Can you work these out from the model? Positions are in its coordinate system, mm. A direction names the side the tool comes from. Round coordinates to 2 decimals unless told otherwise and drop trailing zeros. Loops run counter-clockwise (first coordinate to the right, second up) from the corner with the lowest first, then second, coordinate; pieces in that order, holes last. Notation, with made-up numbers: (76, 34) -> (109, 34) arc R19 cw to (109, 60) -> close; hole circle Ø7 at (-26.75, 6.25). An arc over 180 degrees is marked (long way). Use a Markdown table: item, result.
from build123d import *

# Parameters (mm, degrees)
SKETCH1_W            = 229
SKETCH1_H            = 120
BOSS_EXTRUDE1_DEPTH  = 15
SKETCH2_W            = 20.632503002
SKETCH2_H            = 53.730004003
BOSS_EXTRUDE2_DEPTH  = 15
CUT_EXTRUDE1_REACH   = 239.205
SKETCH3_W            = 61.75
SKETCH3_H            = 25
CUT_EXTRUDE2_REACH   = 239.205
SKETCH4_W            = 61.75
SKETCH4_H            = 25
CUT_EXTRUDE5_REACH   = 239.205
SKETCH10_W           = 61.75
SKETCH10_H           = 25
CUT_EXTRUDE3_REACH   = 239.205
SKETCH5_R            = 7.5
SKETCH9_R            = 6.25
CUT_EXTRUDE4_DEPTH   = 5
LPATTERN2_COUNT      = 4
LPATTERN2_PITCH      = 69.677
LPATTERN2_COUNT_DIR2 = 2
LPATTERN2_PITCH_DIR2 = 100
M5_TAPPED_HOLE1_D    = 4.2
CUT_EXTRUDE6_REACH   = 239.205
SKETCH14_R           = 3.1


with BuildPart() as part:
    # Sketch1 → Boss-Extrude1 (new body)
    with BuildSketch(Plane(origin=(0, 0, 0), x_dir=(1, 0, 0), z_dir=(0, 1, 0))):
        with Locations((-114.5, 0)):
            Rectangle(SKETCH1_W, SKETCH1_H)
    extrude(amount=-BOSS_EXTRUDE1_DEPTH)

    # Sketch2 → Boss-Extrude2 (add)
    with BuildSketch(Plane(origin=(0, 0, 0), x_dir=(1, 0, 0), z_dir=(0, 1, 0))):
        with Locations((10.316251501, 33.134997999)):
            Rectangle(SKETCH2_W, SKETCH2_H)
    extrude(amount=-BOSS_EXTRUDE2_DEPTH)

    # Sketch3 → Cut-Extrude1 (cut, up to next)
    with BuildSketch(Plane(origin=(0, 0, 0), x_dir=(1, 0, 0), z_dir=(0, 1, 0)), mode=Mode.PRIVATE) as cut_extrude1_sk1:
        with Locations((-18.875, 25.846108513)):
            Rectangle(SKETCH3_W, SKETCH3_H)
    cut_extrude1_tool1 = extrude(cut_extrude1_sk1.sketch, amount=-CUT_EXTRUDE1_REACH, mode=Mode.PRIVATE) & part.part
    add(cut_extrude1_tool1.solids().sort_by_distance((-18.875, 0, -25.846109))[0], mode=Mode.SUBTRACT)

    # Sketch4 → Cut-Extrude2 (cut, up to next)
    with BuildSketch(Plane(origin=(0, 0, 0), x_dir=(1, 0, 0), z_dir=(0, 1, 0)), mode=Mode.PRIVATE) as cut_extrude2_sk1:
        with Locations((-98.875, 17.083858316)):
            Rectangle(SKETCH4_W, SKETCH4_H)
    cut_extrude2_tool1 = extrude(cut_extrude2_sk1.sketch, amount=-CUT_EXTRUDE2_REACH, mode=Mode.PRIVATE) & part.part
    add(cut_extrude2_tool1.solids().sort_by_distance((-98.875, 0, -17.083858))[0], mode=Mode.SUBTRACT)

    # Sketch10 → Cut-Extrude5 (cut, up to next)
    with BuildSketch(Plane(origin=(0, 0, 0), x_dir=(1, 0, 0), z_dir=(0, 1, 0)), mode=Mode.PRIVATE) as cut_extrude5_sk1:
        with Locations((-178.875, 16.78)):
            Rectangle(SKETCH10_W, SKETCH10_H)
    cut_extrude5_tool1 = extrude(cut_extrude5_sk1.sketch, amount=-CUT_EXTRUDE5_REACH, mode=Mode.PRIVATE) & part.part
    add(cut_extrude5_tool1.solids().sort_by_distance((-178.875, 0, -16.78))[0], mode=Mode.SUBTRACT)

    # Sketch5 → Cut-Extrude3 (cut, up to next)
    with BuildSketch(Plane(origin=(0, 0, 0), x_dir=(1, 0, 0), z_dir=(0, 1, 0)), mode=Mode.PRIVATE) as cut_extrude3_sk1:
        with Locations(Location((-114.5, 50, 0), (0, 0, 270))):
            Circle(SKETCH5_R)
    cut_extrude3_tool1 = extrude(cut_extrude3_sk1.sketch, amount=-CUT_EXTRUDE3_REACH, mode=Mode.PRIVATE) & part.part
    # Sketch5 → Cut-Extrude3 (cut, up to next)
    with BuildSketch(Plane(origin=(0, 0, 0), x_dir=(1, 0, 0), z_dir=(0, 1, 0)), mode=Mode.PRIVATE) as cut_extrude3_sk2:
        with Locations(Location((-114.5, -50, 0), (0, 0, 270))):
            Circle(SKETCH5_R)
    cut_extrude3_tool2 = extrude(cut_extrude3_sk2.sketch, amount=-CUT_EXTRUDE3_REACH, mode=Mode.PRIVATE) & part.part
    add(cut_extrude3_tool1.solids().sort_by_distance((-114.5, 0, -50))[0], mode=Mode.SUBTRACT)
    add(cut_extrude3_tool2.solids().sort_by_distance((-114.5, 0, 50))[0], mode=Mode.SUBTRACT)

    # Sketch9 → Cut-Extrude4 (cut)
    with BuildSketch(Plane.XZ.offset(15)):
        with Locations(Location((-219, -50, 0), (0, 0, 270))):
            Circle(SKETCH9_R)
    cut_extrude4 = extrude(amount=-CUT_EXTRUDE4_DEPTH, mode=Mode.SUBTRACT)

    # LPattern2: Cut-Extrude4 4 × 2
    with Locations(*[(i * LPATTERN2_PITCH, 0, j * LPATTERN2_PITCH_DIR2) for i in range(LPATTERN2_COUNT) for j in range(LPATTERN2_COUNT_DIR2) if (i, j) != (0, 0)]):
        add(cut_extrude4, mode=Mode.SUBTRACT)

    # M5 Tapped Hole1 (through all)
    with Locations(Plane(origin=(0, -10, 0), x_dir=(-1, 0, 0), z_dir=(0, -1, 0))):
        with Locations((9.969, 50), (219, 50), (219, -50), (9.969, -50)):
            Hole(M5_TAPPED_HOLE1_D / 2)

    # Draft1: read off the stored shape, not the designer's step
    # Draft1: loft between two sections, ruled curve by curve
    draft1_from = [
        Edge.make_line((-50.16206508, 0, -38.758173593), (-50.16206508, 0, -12.934043433)),
        Edge.make_line((12.41206508, 0, -38.758173593), (-50.16206508, 0, -38.758173593)),
        Edge.make_line((12.41206508, 0, -12.934043433), (12.41206508, 0, -38.758173593)),
        Edge.make_line((-50.16206508, 0, -12.934043433), (12.41206508, 0, -12.934043433)),
    ]
    draft1_to = [
        Edge.make_line((-49.75, -11.8, -38.346108513), (-49.75, -11.8, -13.346108513)),
        Edge.make_line((12, -11.8, -38.346108513), (-49.75, -11.8, -38.346108513)),
        Edge.make_line((12, -11.8, -13.346108513), (12, -11.8, -38.346108513)),
        Edge.make_line((-49.75, -11.8, -13.346108513), (12, -11.8, -13.346108513)),
    ]
    draft1 = Solid(Shell([*[Face.make_surface_from_curves(draft1_from[k], draft1_to[k]) for k in range(4)], Face(Wire(draft1_from)), Face(Wire(draft1_to))]))
    add(draft1, mode=Mode.SUBTRACT)

    # Draft1 2: loft between two sections, ruled curve by curve
    draft1_2_from = [
        Edge.make_line((-130.16206508, 0, -29.995923396), (-130.16206508, 0, -4.171793236)),
        Edge.make_line((-67.58793492, 0, -29.995923396), (-130.16206508, 0, -29.995923396)),
        Edge.make_line((-67.58793492, 0, -4.171793236), (-67.58793492, 0, -29.995923396)),
        Edge.make_line((-130.16206508, 0, -4.171793236), (-67.58793492, 0, -4.171793236)),
    ]
    draft1_2_to = [
        Edge.make_line((-129.75, -11.8, -29.583858316), (-129.75, -11.8, -4.583858316)),
        Edge.make_line((-68, -11.8, -29.583858316), (-129.75, -11.8, -29.583858316)),
        Edge.make_line((-68, -11.8, -4.583858316), (-68, -11.8, -29.583858316)),
        Edge.make_line((-129.75, -11.8, -4.583858316), (-68, -11.8, -4.583858316)),
    ]
    draft1_2 = Solid(Shell([*[Face.make_surface_from_curves(draft1_2_from[k], draft1_2_to[k]) for k in range(4)], Face(Wire(draft1_2_from)), Face(Wire(draft1_2_to))]))
    add(draft1_2, mode=Mode.SUBTRACT)

    # Draft1 3: loft between two sections, ruled curve by curve
    draft1_3_from = [
        Edge.make_line((-210.16206508, 0, -29.69206508), (-210.16206508, 0, -3.86793492)),
        Edge.make_line((-147.58793492, 0, -29.69206508), (-210.16206508, 0, -29.69206508)),
        Edge.make_line((-147.58793492, 0, -3.86793492), (-147.58793492, 0, -29.69206508)),
        Edge.make_line((-210.16206508, 0, -3.86793492), (-147.58793492, 0, -3.86793492)),
    ]
    draft1_3_to = [
        Edge.make_line((-209.75, -11.8, -29.28), (-209.75, -11.8, -4.28)),
        Edge.make_line((-148, -11.8, -29.28), (-209.75, -11.8, -29.28)),
        Edge.make_line((-148, -11.8, -4.28), (-148, -11.8, -29.28)),
        Edge.make_line((-209.75, -11.8, -4.28), (-148, -11.8, -4.28)),
    ]
    draft1_3 = Solid(Shell([*[Face.make_surface_from_curves(draft1_3_from[k], draft1_3_to[k]) for k in range(4)], Face(Wire(draft1_3_from)), Face(Wire(draft1_3_to))]))
    add(draft1_3, mode=Mode.SUBTRACT)

    # Sketch14 → Cut-Extrude6 (cut, up to next)
    with BuildSketch(Plane(origin=(0, 0, 0), x_dir=(1, 0, 0), z_dir=(0, 1, 0)), mode=Mode.PRIVATE) as cut_extrude6_sk1:
        with Locations(Location((-179, -14.72, 0), (0, 0, 270))):
            Circle(SKETCH14_R)
    cut_extrude6_tool1 = extrude(cut_extrude6_sk1.sketch, amount=-CUT_EXTRUDE6_REACH, mode=Mode.PRIVATE) & part.part
    # Sketch14 → Cut-Extrude6 (cut, up to next)
    with BuildSketch(Plane(origin=(0, 0, 0), x_dir=(1, 0, 0), z_dir=(0, 1, 0)), mode=Mode.PRIVATE) as cut_extrude6_sk2:
        with Locations(Location((-139, -14.72, 0), (0, 0, 270))):
            Circle(SKETCH14_R)
    cut_extrude6_tool2 = extrude(cut_extrude6_sk2.sketch, amount=-CUT_EXTRUDE6_REACH, mode=Mode.PRIVATE) & part.part
    # Sketch14 → Cut-Extrude6 (cut, up to next)
    with BuildSketch(Plane(origin=(0, 0, 0), x_dir=(1, 0, 0), z_dir=(0, 1, 0)), mode=Mode.PRIVATE) as cut_extrude6_sk3:
        with Locations(Location((-99, -14.72, 0), (0, 0, 270))):
            Circle(SKETCH14_R)
    cut_extrude6_tool3 = extrude(cut_extrude6_sk3.sketch, amount=-CUT_EXTRUDE6_REACH, mode=Mode.PRIVATE) & part.part
    # Sketch14 → Cut-Extrude6 (cut, up to next)
    with BuildSketch(Plane(origin=(0, 0, 0), x_dir=(1, 0, 0), z_dir=(0, 1, 0)), mode=Mode.PRIVATE) as cut_extrude6_sk4:
        with Locations(Location((-59, -14.72, 0), (0, 0, 270))):
            Circle(SKETCH14_R)
    cut_extrude6_tool4 = extrude(cut_extrude6_sk4.sketch, amount=-CUT_EXTRUDE6_REACH, mode=Mode.PRIVATE) & part.part
    # Sketch14 → Cut-Extrude6 (cut, up to next)
    with BuildSketch(Plane(origin=(0, 0, 0), x_dir=(1, 0, 0), z_dir=(0, 1, 0)), mode=Mode.PRIVATE) as cut_extrude6_sk5:
        with Locations(Location((-19, -14.72, 0), (0, 0, 270))):
            Circle(SKETCH14_R)
    cut_extrude6_tool5 = extrude(cut_extrude6_sk5.sketch, amount=-CUT_EXTRUDE6_REACH, mode=Mode.PRIVATE) & part.part
    add(cut_extrude6_tool1.solids().sort_by_distance((-179, 0, 14.72))[0], mode=Mode.SUBTRACT)
    add(cut_extrude6_tool2.solids().sort_by_distance((-139, 0, 14.72))[0], mode=Mode.SUBTRACT)
    add(cut_extrude6_tool3.solids().sort_by_distance((-99, 0, 14.72))[0], mode=Mode.SUBTRACT)
    add(cut_extrude6_tool4.solids().sort_by_distance((-59, 0, 14.72))[0], mode=Mode.SUBTRACT)
    add(cut_extrude6_tool5.solids().sort_by_distance((-19, 0, 14.72))[0], mode=Mode.SUBTRACT)


solid = part.part
1. Which directions (+Z, -Z, +X, -X, +Y, -Y) give clear straight access to the entire face, cutting with the end or side of a thin tool? Please do faces 3 (the flat face through (0, -7, 27)), 4 (the flat face through (-149, -10, 50)), 5 (the cylindrical face through (-55.926, -7.395, 14.316)).
Answer sheet:
| item | result |
|---|---|
| face 3 | +Z, +X, +Y, -Y |
| face 4 | -Y |
| face 5 | +Y, -Y |
2. I want a section at D-D (z = 39). Please give me the cut outline in (x, y).
Answer sheet:
| item | result |
|---|---|
| outline | (-229, -15) -> (0, -15) -> (0, 0) -> (-229, 0) -> close |
3. If we mould it in two halves opening along Z, with no side actions, what happens to faces 1 (the cylindrical face through (-220.666, -4.93, -48.722)), 2 (the flat face through (-106, 0, -1))? For each: +Z half, -Z half, draft (parallel to the pull), parting line (faces both ways), or undercut.
Answer sheet:
| item | result |
|---|---|
| face 1 | undercut |
| face 2 | draft |
4. I need wall thicknesses on line 1 (Z direction, x = -80, y = -11.25); line 2 (X direction, y = -11.55, z = 50); line 3 (Z direction, x = -139, y = -11.75). Which ranges of each line are inside material? Lowest first, please.
Answer sheet:
| item | result |
|---|---|
| line 1 | z = -60 to -56.24, -43.76 to -29.6, -4.56 to 43.76, 56.24 to 60 |
| line 2 | x = -229 to -225.25, -212.75 to -155.57, -143.07 to -122, -107 to -85.9, -73.4 to -16.22, -3.72 to 0 |
| line 3 | z = -60 to 11.62, 17.82 to 60 |
5. I want a section at C-C (y = -4). State how many separate pieces and enclosed holes the cut face has, plus the area to 3 significant figures.
Answer sheet:
| item | result |
|---|---|
| separate pieces | 1 |
| enclosed holes | 14 |
| area | 23,300 mm² |
6. Will these pins go through, and if not, where does the flat tip stop? pin 1 Ø4 at (x, z) = (-80.5, -51) entering from -Y; pin 2 Ø13.5 at (x, z) = (-114.5, 50) entering from -Y.
Answer sheet:
| item | result |
|---|---|
| pin 1 | stops at y = -10 |
| pin 2 | passes through |
7. I want a section at A-A (x = -59). Please give me the cut outline in (y, z).
Answer sheet:
| item | result |
|---|---|
| outline | (-15, -60) -> (0, -60) -> (0, 11.62) -> (-15, 11.62) -> close; (-15, 17.82) -> (0, 17.82) -> (0, 60) -> (-15, 60) -> close |
8. I want a section at B-B (z = 14). Please give me the cut outline in (x, y).
Answer sheet:
| item | result |
|---|---|
| outline | (-229, -15) -> (-182.02, -15) -> (-182.02, 0) -> (-229, 0) -> close; (-175.98, -15) -> (-142.02, -15) -> (-142.02, 0) -> (-175.98, 0) -> close; (-135.98, -15) -> (-102.02, -15) -> (-102.02, 0) -> (-135.98, 0) -> close; (-95.98, -15) -> (-62.02, -15) -> (-62.02, 0) -> (-95.98, 0) -> close; (-55.98, -15) -> (-22.02, -15) -> (-22.02, 0) -> (-55.98, 0) -> close; (-15.98, -15) -> (0, -15) -> (0, 0) -> (-15.98, 0) -> close |
